The drawing under review shows one solid part. Ordinate dimensions are in mm from its lowest x, y, z. Give positions to 0.01 mm unless a question says otherwise; leave off trailing zeros. Write each loop counter-clockwise with the first axis right and the second up, starting at its lowest first coordinate (ties: lowest second). Pieces come first, ordered by that corner, then holes.
Q1. We need section D-D (x = 16). Write out the cut boundary in (y, z).
Q2. For line 1 (X direction, y = 30, z = 45); line 2 (X direction, y = 24, z = 40); line 3 (Z direction, x = 27.5, y = 28.5), list the stretches that pass through material, from the lowest coordinate up.
Q3. We need section B-B (z = 40.5). Write out the cut boundary in (x, y), then the cut area to 3 significant figures.
Q4. We need section C-C (x = 24). Write out the cut boundary in (y, z), then the cut area to 3 significant figures.
Q5. We need section A-A (y = 8.5). Write out the cut boundary in (x, z).
Q6. Mouldability with a two-part tool opening along X and no side actions: class the marked faces 1, 2 and 3 as released by +X, released by -X, zero draft, split by the parting line, or undercut.
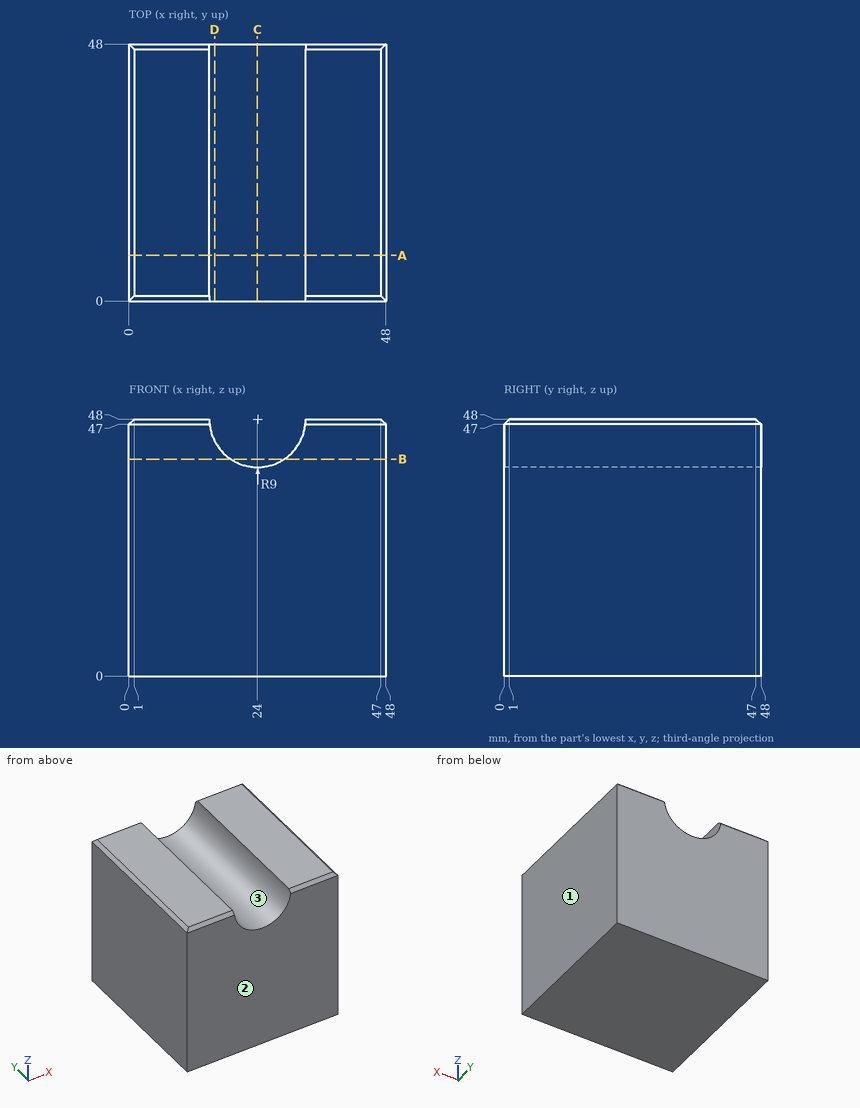
Computed:
1. outline: (0, 0) - (48, 0) - (48, 43.88) - (0, 43.88) - close
2. line 1: x = 0 to 15.51, 32.49 to 48
2. line 2: x = 0 to 19.88, 28.12 to 48
2. line 3: z = 0 to 39.71
3. outline: (0, 0) - (19.03, 0) - (19.03, 48) - (0, 48) - close; (28.97, 0) - (48, 0) - (48, 48) - (28.97, 48) - close
3. area: 1,830 mm2
4. outline: (0, 0) - (48, 0) - (48, 39) - (0, 39) - close
4. area: 1,870 mm2
5. outline: (0, 0) - (48, 0) - (48, 47) - (47, 48) - (33, 48) arc R9 cw to (15, 48) - (1, 48) - (0, 47) - close
6. face 1: released by +X
6. face 2: zero draft
6. face 3: undercut
